Work out the finished part from the listing and answer in its coordinate system (mm). Round coordinates to 2 decimals unless told otherwise and drop trailing zeros. Write each loop counter-clockwise with the first axis right and the second up, starting at its lowest first coordinate (ties: lowest second). Pieces come first, ordered by that corner, then holes. Notation, with made-up numbers: M 54,89 L 70,89 A29 cw 70,120 Z; hole C 65.25,-37 d6. An arc over 180 degrees is marked long. One line per item, written item: value. Start each with the question number.
Q1. Consider probe 1 along Z at (x, y) = (-30.25, 41.25); probe 2 along Y at (x, z) = (-24.25, 0.45); probe 3 along X at (y, z) = (31, 0.1). Determine where each line is inside the solid, lowest interval first.
Q2. Find section B-B (z = 0.25). Write down the section's boundary in (x, y), and give its area (3 significant figures).
Q3. Find section C-C (z = 1.3). Write down the section's boundary in (x, y), and give its area (3 significant figures).
from build123d import *

# Parameters (mm, degrees)
F0_W     = 13
F0_H     = 18
F1_DEPTH = 1
F2_R     = 5.5
F3_DEPTH = 0.5
F4_R     = 0.49999


# Not quite as in the source:
# - a fillet or chamfer is up to 0.001 mm smaller than in the source, because OpenCascade refuses the exact size


with BuildPart() as f1:
    # F0 (on Top) → F1 (new body)
    with BuildSketch(Plane.XY):
        with Locations((-28.8841596369, 33.0711239949)):
            Rectangle(F0_W, F0_H)
    extrude(amount=F1_DEPTH)

    # F2 (on face) → F3 (join)
    with BuildSketch(Plane.XY.offset(1)):
        with Locations((-28.8841596369, 33.0711239949)):
            Circle(F2_R)
    extrude(amount=F3_DEPTH)

    # F4 (radius 0.5 in the source; OpenCascade refuses exactly that, so slightly less here)
    f4_edges = [f1.edges().sort_by_distance(p)[0] for p in [
        (-28.88416, 42.071124, 1),
        (-28.88416, 42.071124, 0),
        (-35.38416, 33.071124, 1),
        (-22.38416, 33.071124, 1),
        (-28.88416, 24.071124, 1),
        (-34.38416, 33.071124, 1.5),
        (-22.38416, 42.071124, 0.5),
        (-22.38416, 33.071124, 0),
        (-35.38416, 33.071124, 0),
        (-28.88416, 24.071124, 0),
        (-22.38416, 24.071124, 0.5),
        (-35.38416, 24.071124, 0.5),
        (-35.38416, 42.071124, 0.5),
    ]]
    fillet(f4_edges, radius=F4_R)


solid = f1.part
The answers:
1. probe 1: 0 to 1
1. probe 2: 24.07 to 42.07
1. probe 3: -35.18 to -22.58
2. outline: M -35.32,24.57 A0.43 ccw -34.88,24.14 L -22.88,24.14 A0.43 ccw -22.45,24.57 L -22.45,41.57 A0.43 ccw -22.88,42 L -34.88,42 A0.43 ccw -35.32,41.57 Z
2. area: 230 mm2
3. outline: C -28.88,33.07 d10.8
3. area: 91.6 mm2
